from build123d import *
from OCP.BRepFilletAPI import BRepFilletAPI_MakeChamfer

# Parameters (mm, degrees)
SKETCH1_W               = 95.25
SKETCH1_H               = 95.25
BOSS_EXTRUDE1_DEPTH     = 19.05
CUT_EXTRUDE1_DEPTH      = 6.35
LEGS_OUTER_SIZE         = 2.54
TOP_FACE_SIZE           = 1.27
LEGS_INNER_SIZE         = 1.016
CUT_EXTRUDE5_DEPTH      = 69.538830235
CUT_EXTRUDE5_DEPTH_BACK = 11.684
SKETCH6_W               = 82.55
SKETCH6_H               = 82.55
SKETCH3_3_W             = 69.85
SKETCH3_3_H             = 69.85
CUT_EXTRUDE6_DEPTH      = 70.9941694
CHAMFER3_SIZE           = 0.381
CHAMFER3_SIZE2          = 0.659911358
CUT_EXTRUDE3_DEPTH      = 18.034


with BuildPart() as part:
    # Sketch1 → Boss-Extrude1 (new body)
    with BuildSketch(Plane(origin=(0, 0, 0), x_dir=(1, 0, 0), z_dir=(0, 1, 0))):
        Rectangle(SKETCH1_W, SKETCH1_H)
    extrude(amount=BOSS_EXTRUDE1_DEPTH)

    # Sketch1<3> → Cut-Extrude1 (cut)
    with BuildSketch(Plane(origin=(0, 0, 0), x_dir=(1, 0, 0), z_dir=(0, 1, 0))):
        Polygon((-47.625, -34.925), (-34.925, -34.925), (-34.925, -47.625), (34.925, -47.625), (34.925, -34.925), (47.625, -34.925), (47.625, 34.925), (34.925, 34.925), (34.925, 47.625), (-34.925, 47.625), (-34.925, 34.925), (-47.625, 34.925), align=None)
    extrude(amount=CUT_EXTRUDE1_DEPTH, mode=Mode.SUBTRACT)

    # legs, outer
    legs_outer_edges = [part.edges().sort_by_distance(p)[0] for p in [
        (-47.625, 9.525, 47.625),
        (47.625, 9.525, 47.625),
        (47.625, 9.525, -47.625),
        (-47.625, 9.525, -47.625),
    ]]
    chamfer(legs_outer_edges, length=LEGS_OUTER_SIZE)

    # top face
    top_face_edges = [part.edges().sort_by_distance(p)[0] for p in [
        (0, 19.05, -47.625),
        (47.625, 19.05, 0),
        (-47.625, 19.05, 0),
        (0, 19.05, 47.625),
        (-46.355, 19.05, -46.355),
        (-46.355, 19.05, 46.355),
        (46.355, 19.05, 46.355),
        (46.355, 19.05, -46.355),
    ]]
    chamfer(top_face_edges, length=TOP_FACE_SIZE)

    # legs, inner
    legs_inner_edges = [part.edges().sort_by_distance(p)[0] for p in [
        (-47.625, 3.175, 34.925),
        (-47.625, 3.175, -34.925),
        (-34.925, 3.175, -47.625),
        (34.925, 3.175, -47.625),
        (47.625, 3.175, -34.925),
        (47.625, 3.175, 34.925),
        (34.925, 3.175, 47.625),
        (-34.925, 3.175, 47.625),
    ]]
    chamfer(legs_inner_edges, length=LEGS_INNER_SIZE)

    # Sketch6 → Cut-Extrude5 (cut, two sides: drawn at the far end of the back side and taken through both)
    with BuildSketch(Plane.XZ.offset(-6.35).offset(-CUT_EXTRUDE5_DEPTH_BACK)):
        Rectangle(SKETCH6_W, SKETCH6_H)
    extrude(amount=CUT_EXTRUDE5_DEPTH + CUT_EXTRUDE5_DEPTH_BACK, mode=Mode.SUBTRACT)

    # Sketch3<3> → Cut-Extrude6 (cut, through all)
    with BuildSketch(Plane(origin=(0, 0, 0), x_dir=(1, 0, 0), z_dir=(0, 1, 0))):
        Rectangle(SKETCH3_3_W, SKETCH3_3_H)
    extrude(amount=CUT_EXTRUDE6_DEPTH, mode=Mode.SUBTRACT)

    # Chamfer3: one chamfer whose edges measure the first distance from different faces: ONE call of the kernel's chamfer builder (chamfer() names one face for all edges)
    chamfer3_edges_1 = [part.edges().sort_by_distance(p)[0] for p in [
        (34.925, 19.05, 0),
    ]]
    chamfer3_side_1 = [part.faces().sort_by_distance(p)[0] for p in [
        (34.925, 18.542, 0),
    ]]
    chamfer3_edges_2 = [part.edges().sort_by_distance(p)[0] for p in [
        (0, 19.05, -34.925),
    ]]
    chamfer3_side_2 = [part.faces().sort_by_distance(p)[0] for p in [
        (0, 18.542, -34.925),
    ]]
    chamfer3_edges_3 = [part.edges().sort_by_distance(p)[0] for p in [
        (-34.925, 19.05, 0),
    ]]
    chamfer3_side_3 = [part.faces().sort_by_distance(p)[0] for p in [
        (-34.925, 18.542, 0),
    ]]
    chamfer3_edges_4 = [part.edges().sort_by_distance(p)[0] for p in [
        (0, 19.05, 34.925),
    ]]
    chamfer3_side_4 = [part.faces().sort_by_distance(p)[0] for p in [
        (0, 18.542, 34.925),
    ]]
    chamfer3 = BRepFilletAPI_MakeChamfer(part.part.solid().wrapped)
    for e in chamfer3_edges_1:
        chamfer3.Add(CHAMFER3_SIZE, CHAMFER3_SIZE2, e.wrapped, chamfer3_side_1[0].wrapped)  # the first distance lies on this face
    for e in chamfer3_edges_2:
        chamfer3.Add(CHAMFER3_SIZE, CHAMFER3_SIZE2, e.wrapped, chamfer3_side_2[0].wrapped)  # the first distance lies on this face
    for e in chamfer3_edges_3:
        chamfer3.Add(CHAMFER3_SIZE, CHAMFER3_SIZE2, e.wrapped, chamfer3_side_3[0].wrapped)  # the first distance lies on this face
    for e in chamfer3_edges_4:
        chamfer3.Add(CHAMFER3_SIZE, CHAMFER3_SIZE2, e.wrapped, chamfer3_side_4[0].wrapped)  # the first distance lies on this face
    add(Compound.cast(chamfer3.Shape()), mode=Mode.REPLACE)

    # Sketch3 → Cut-Extrude3 (cut)
    with BuildSketch(Plane(origin=(0, 0, 0), x_dir=(1, 0, 0), z_dir=(0, 1, 0))):
        with BuildLine():
            ThreePointArc((37.592, 40.767), (38.52193597, 38.52193597), (40.767, 37.592))
            Line((40.767, 37.592), (40.767, 40.767))
            Line((40.767, 40.767), (37.592, 40.767))
        make_face()
        with BuildLine():
            Line((40.767, 40.767), (40.767, 37.592))
            ThreePointArc((40.767, 37.592), (43.01206403, 38.52193597), (43.942, 40.767))
            ThreePointArc((43.942, 40.767), (40.767, 43.942), (37.592, 40.767))
            Line((37.592, 40.767), (40.767, 40.767))
        make_face()
        with BuildLine():
            ThreePointArc((-37.592, 40.767), (-43.01206403, 43.01206403), (-40.767, 37.592))
            Line((-40.767, 37.592), (-40.767, 40.767))
            Line((-40.767, 40.767), (-37.592, 40.767))
        make_face()
        with BuildLine():
            Line((-40.767, 40.767), (-40.767, 37.592))
            ThreePointArc((-40.767, 37.592), (-38.52193597, 38.52193597), (-37.592, 40.767))
            Line((-37.592, 40.767), (-40.767, 40.767))
        make_face()
        with BuildLine():
            ThreePointArc((40.767, -37.592), (38.52193597, -38.52193597), (37.592, -40.767))
            Line((37.592, -40.767), (40.767, -40.767))
            Line((40.767, -40.767), (40.767, -37.592))
        make_face()
        with BuildLine():
            Line((40.767, -40.767), (37.592, -40.767))
            ThreePointArc((37.592, -40.767), (40.767, -43.942), (43.942, -40.767))
            ThreePointArc((43.942, -40.767), (43.01206403, -38.52193597), (40.767, -37.592))
            Line((40.767, -37.592), (40.767, -40.767))
        make_face()
        with BuildLine():
            Line((-40.767, -37.592), (-40.767, -40.767))
            Line((-40.767, -40.767), (-37.592, -40.767))
            ThreePointArc((-37.592, -40.767), (-38.52193597, -38.52193597), (-40.767, -37.592))
        make_face()
        with BuildLine():
            Line((-37.592, -40.767), (-40.767, -40.767))
            Line((-40.767, -40.767), (-40.767, -37.592))
            ThreePointArc((-40.767, -37.592), (-43.01206403, -43.01206403), (-37.592, -40.767))
        make_face()
    extrude(amount=CUT_EXTRUDE3_DEPTH, mode=Mode.SUBTRACT)


solid = part.part
Input: part model. Units: mm. Frame: model coordinates. A direction names the side the tool comes from. Give positions to 0.01 mm unless a question says otherwise; leave off trailing zeros. Loops run counter-clockwise (first coordinate to the right, second up) from the corner with the lowest first, then second, coordinate; pieces in that order, holes last. Notation, with made-up numbers: M 84.5,48.25 L 105.5,48.25 A23 cw 105.5,85.25 Z; hole C 36,-18.75 d11. An arc over 180 degrees is marked long. Use one line per item in the form item = value.
1. Section query B-B, the plane y = 8.5. Return the cut outline in (x, z) (3 decimals), and give its area (3 significant figures).
Numbers:
outline = M -47.625,-45.085 L -45.085,-47.625 L 45.085,-47.625 L 47.625,-45.085 L 47.625,45.085 L 45.085,47.625 L -45.085,47.625 L -47.625,45.085 Z; hole M -41.275,-37.633 A3.175 ccw long -37.633,-41.275 L 37.633,-41.275 A3.175 ccw long 41.275,-37.633 L 41.275,37.633 A3.175 ccw long 37.633,41.275 L -37.633,41.275 A3.175 ccw long -41.275,37.633 Z
area = 2,160 mm²
2. Reachability of faces 5 (the face through (-1, 11, -41.275)), 6 (the face through (-34.925, 3, -44)), 7 (the face through (-44, 3, -34.925)), 8 (the face through (47.625, 11, 1)) from +Z, -Z, +X, -X, +Y, -Y: full face, straight path, thin tool, end or side. Return the list, or none.
Numbers:
face_5 = -Y
face_6 = +Z, -Z, -Y
face_7 = +X, -X, -Y
face_8 = +Z, -Z, +X, +Y, -Y
3. Pull-direction query (Z, two-part tool) for faces 1 (the face through (-41.275, 11, -1)), 2 (the face through (46.37, 8.77, -46.34)), 3 (the face through (-45.917, 18.424, 45.882)), 4 (the face through (-1, 6.35, 44)); classes: released by +Z, released by -Z, zero draft, split by the parting line, or undercut.
Numbers:
face_1 = undercut
face_2 = released by -Z
face_3 = released by +Z
face_4 = zero draft
4. First-contact query: pin 1 (7 mm diameter, centred on x = -8.5, z = -45, fed in from -Y); pin 2 (2 mm diameter, centred on x = -8, z = 34.5, fed in from -Y); pin 3 (0.5 mm diameter, centred on x = 2, y = 18.5, fed in from -Z) (3 decimals). Flat tips, straight axial feed; report the tip coordinate or a pass-through.
Numbers:
pin_1 = 6.35
pin_2 = 18.03
pin_3 = -47.155
5. Line query: L1, parallel to X at y = 17.25, z = 3 (3 decimals); L2, parallel to Z at x = 42.5, y = 14.5 (3 decimals). Output: solid intervals per line, ascending.
Numbers:
L1 = -47.625 to -41.275, 41.275 to 47.625
L2 = -47.625 to -43.427, -38.107 to 38.107, 43.427 to 47.625
6. Section query C-C, the plane x = -2. Return the cut outline in (y, z) (3 decimals), and give its area (3 significant figures).
Numbers:
outline = M 6.35,-47.625 L 17.78,-47.625 L 19.05,-46.355 L 19.05,-35.585 L 18.669,-34.925 L 18.034,-34.925 L 18.034,-41.275 L 6.35,-41.275 Z; M 6.35,41.275 L 18.034,41.275 L 18.034,34.925 L 18.669,34.925 L 19.05,35.585 L 19.05,46.355 L 17.78,47.625 L 6.35,47.625 Z
area = 172 mm²
7. Section query D-D, the plane x = -40. Return the cut outline in (y, z) (3 decimals).
Numbers:
outline = M 0,-47.625 L 17.78,-47.625 L 19.05,-46.355 L 19.05,46.355 L 17.78,47.625 L 0,47.625 L 0,43.848 L 18.034,43.848 L 18.034,-43.848 L 0,-43.848 Z
8. Section query A-A, the plane z = -27. Return the cut outline in (x, y) (3 decimals), and give its area (3 significant figures).
Numbers:
outline = M -47.625,6.35 L -41.275,6.35 L -41.275,18.034 L -34.925,18.034 L -34.925,18.669 L -35.585,19.05 L -46.355,19.05 L -47.625,17.78 Z; M 34.925,18.034 L 41.275,18.034 L 41.275,6.35 L 47.625,6.35 L 47.625,17.78 L 46.355,19.05 L 35.585,19.05 L 34.925,18.669 Z
area = 172 mm²
